Can you work these out from the model? Positions are in its coordinate system, mm. Face numbers are marked on the shaded views. A direction names the side the tool comes from. Give positions to 0.01 mm unless a question says otherwise; leave off trailing zeros. Loops run counter-clockwise (first coordinate to the right, second up) from the corner with the lowest first, then second, coordinate; pieces in that order, holes last. Notation, with made-up numbers: M -17,45.5 L -2,45.5 A18 ccw -2,67.5 Z; hole C 22.25,49 d1. An arc over 180 degrees is marked long. Use CSV: the item, a comma, the result in double quotes.
Autodesk Inventor part; units mm, degrees
ref_plane "Work Plane2" through (3.35, 0, 0) normal (0, 0, -1) x (1, 0, 0)
ref_plane "YZ Plane" through (0, 0, 0) normal (1, 0, 0) x (0, 1, 0)
ref_plane "XZ Plane" through (0, 0, 0) normal (0, 1, 0) x (-1, 0, 0)
sketch "Sketch1" plane through (0, 0, 0) normal (0, 0, 1) x (1, 0, 0)
  line L0 (1.88, 0) -> (8, 0)
  line L1 (8, 0) -> (8, 2)
  line L2 (8, 2) -> (3.6, 2)
  line L3 (3.6, 2) -> (3.1706, 1.7853)
  line L4 (3.1706, 1.7853) -> (2.2, 1.7853)
  line L5 (0, 3.5) -> (0, 2.11)
  line L6 (0, 2.11) -> (1.0316, 1.5957)
  line L7 (1.0316, 1.5957) -> (1.88, 0)
  line L8 (-1.6, 0) -> (9.6, 0)
  line L9 (0, -0.7) -> (0, 4.2)
  line L10 (0, 3.5) -> (0.4853, 3.5)
  line L11 (0.4853, 3.5) -> (2.2, 1.7853)
  line L12 (3.6, 2) -> (1.9853, 2) construction
  dimension "d1" = 4.4
  dimension "d2" = 4
  dimension "d3" = 3.5706
  dimension "d4" = 4.22
  dimension "d5" = 26.5
  dimension "d6" = 62
  dimension "d7" = 1.88
  dimension "d8" = 0.4294
  dimension "d12" = 7
  dimension "d13" = 45
  dimension "d15" = 8
  dimension "d24" = 2.2
revolve "Body" add sketch "Sketch1" angle 360 about axis through (1.88, 0, 0) along (1, 0, 0) contours L7 L6 L5 L10 L11 L4 L3 L2 L1 L0
sketch "Sketch2" plane through (0, 0, 0) normal (-1, 0, 0) x (0, 0, 1)
  line L0 (0, 2.11) -> (0, 0) construction
  line L1 (0, 0) -> (2.11, 0) construction
  arc A0 (0.633, 0) -> (0, 0.633) centre (0, 0) ccw construction
  arc A1 (0.7385, 0) -> (0, 0.7385) centre (0, 0) ccw construction
  arc A2 (2.0511, 0.495) -> (0.495, 2.0511) centre (0, 0) ccw
  line L2 (0, 0) -> (1.492, 1.492) construction
  line L3 (0.495, 2.0511) -> (0.3793, 0.6337)
  line L4 (2.0511, 0.495) -> (0.6337, 0.3793)
  arc A3 (0.495, 2.0511) -> (0, 2.11) centre (0, 0) ccw
  arc A4 (2.11, 0) -> (2.0511, 0.495) centre (0, 0) ccw
  line L5 (0, -4.9) -> (0, 4.9)
  line L6 (-4.9, 0) -> (4.9, 0)
  arc A5 (0.495, -2.0511) -> (2.0511, -0.495) centre (0, 0) ccw
  line L7 (0.495, -2.0511) -> (0.3793, -0.6337)
  line L8 (2.0511, -0.495) -> (0.6337, -0.3793)
  arc A6 (0, -2.11) -> (0.495, -2.0511) centre (0, 0) ccw
  arc A7 (2.0511, -0.495) -> (2.11, 0) centre (0, 0) ccw
  arc A8 (-0.495, 2.0511) -> (-2.0511, 0.495) centre (0, 0) ccw
  line L9 (-0.495, 2.0511) -> (-0.3793, 0.6337)
  line L10 (-2.0511, 0.495) -> (-0.6337, 0.3793)
  arc A9 (0, 2.11) -> (-0.495, 2.0511) centre (0, 0) ccw
  arc A10 (-2.0511, 0.495) -> (-2.11, 0) centre (0, 0) ccw
  arc A11 (-0.495, -2.0511) -> (0, -2.11) centre (0, 0) ccw
  arc A12 (-2.0511, -0.495) -> (-0.495, -2.0511) centre (0, 0) ccw
  arc A13 (-2.11, 0) -> (-2.0511, -0.495) centre (0, 0) ccw
  line L11 (-2.0511, -0.495) -> (-0.6337, -0.3793)
  line L12 (-0.495, -2.0511) -> (-0.3793, -0.6337)
  arc A14 (0.3793, 0.6337) -> (0.6337, 0.3793) centre (0.6145, 0.6145) ccw
  arc A15 (0.6337, -0.3793) -> (0.3793, -0.6337) centre (0.6145, -0.6145) ccw
  arc A16 (-0.6337, 0.3793) -> (-0.3793, 0.6337) centre (-0.6145, 0.6145) ccw
  arc A17 (-0.3793, -0.6337) -> (-0.6337, -0.3793) centre (-0.6145, -0.6145) ccw
  point P0 (1.492, -1.492)
  point P1 (-1.492, 1.492)
  point P2 (-1.492, -1.492)
  dimension "d17" = 1.266
  dimension "d18" = 1.477
  dimension "d19" = 4.22
  dimension "d20" = 45
  dimension "d21" = 0.495
extrude "Slot" add sketch "Sketch2" against normal up to next draft 5 contours L4 A14 L3 A2 | A5 L7 A15 L8 | L9 A16 L10 A8 | A12 L11 A17 L12
fillet "Fillet1" radius 0.198 4 edges at (0, 2.11, 0) (0, 0, -2.11) (0, -2.11, 0) (0, 0, 2.11)
thread "Thread"
chamfer "Chamfer1" distance 0.4294 distance2 0.2147 1 edges at (8, -2, 0) measured on face at (8, -0.499, 0.4421)
ref_plane "Work Plane2" through (3.35, 0, 0) normal (0, 0, -1) x (1, 0, 0)
equation "\"d17\" = 0.3 * SDM"
equation "\"d18\" = 0.35 * SDM"
equation "\"d19\" = SDM"
equation "\"d21\" = 0.5 * SBR"
equation "\"d1\" = GEL"
equation "\"d2\" = GD"
equation "\"d3\" = BDM"
equation "\"d4\" = SDM"
equation "\"d7\" = INTI"
equation "\"d8\" = GAL"
equation "\"d12\" = KOD"
equation "\"d13\" = 0.5 * SEWI"
equation "\"d15\" = NLG"
equation "\"d24\" = KOH"
equation "\"d23\" = 0.2 * SBR"
equation "\"d10\" = GEL"
equation "\"d25\" = -0.5 * SPD + 0.5 * GD"
equation "\"d26\" = 0.5 * GAL"
equation "\"NLG\" = 8"
equation "\"GEL\" = 4.4"
equation "\"GAL\" = 0.61345 * PTC"
equation "\"SPD\" = NND - 1.2269 * PTC"
equation "\"KOD\" = 7"
equation "\"KOH\" = 2.2"
equation "\"SBR\" = 0.99"
equation "\"INTI\" = 1.88"
equation "\"SDM\" = 4.22"
equation "\"GD\" = NND"
equation "\"BDM\" = NND - GAL"
equation "\"SEWI\" = 90deg"
equation "\"d9\" = SDM"
equation "\"GUL\" = 0.61345 * PTC"
equation "\"TOA\" = 30deg"
equation "\"EPV\" = 4.2"
equation "\"THREADDIA\" = 4"
equation "\"RR\" = 0.4"
equation "\"PTC\" = 0.7"
equation "\"NND\" = 4"
equation "\"GD1\" = THREADDIA - 1.2269 * PTC"
properties part number "AS 1427 - M4 x 8" material "Steel, Mild"
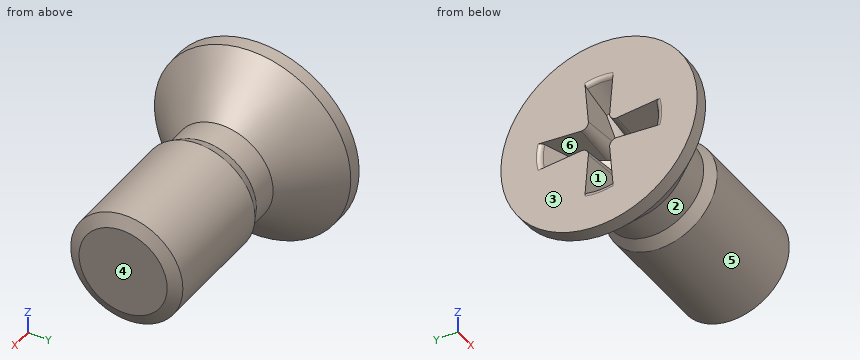
Q1. I want a section at B-B, the plane x = 2.75. Please give me the cut outline in (y, z), then the cut area to 3 significant figures.
Model answer:
outline,"C 0,0 d3.57"
area,"10.0 mm2"
Q2. Please list where these lines run through material, in increasing order: L1, parallel to Y at x = 1.25, z = -0.75; L2, parallel to Z at x = 3.75, y = 0; L3, parallel to Z at x = 0.5, y = 1. Write a range as from..to.
Model answer:
L1,"-2.63..-0.28, 0.28..2.63"
L2,"-2..2"
L3,"-3.34..-0.37, 0.37..3.34"
Q3. If we mould it in two halves opening along Z, with no side actions, what happens to the marked faces 1, 2 and 3? For each: released by +Z, released by -Z, zero draft, split by the parting line, or undercut.
Model answer:
face 1,"undercut"
face 2,"split by the parting line"
face 3,"zero draft"
Q4. I want a section at A-A, the plane x = 5.5. Please give me the cut outline in (y, z), then the cut area to 3 significant figures.
Model answer:
outline,"C 0,0 d4"
area,"12.6 mm2"
Q5. I'm going to push flat-ended pins straight in: P1, Ø1.5, axis at y = 2, z = 0, coming from the +X side; P2, Ø1.5, axis at y = 2, z = -2.5, coming from the +X side; P3, Ø1.5, axis at x = 4.5, z = 1, coming from the +Y side; P4, Ø1.5, axis at x = 2, y = -0.5, coming from the +Z side. Where does each tip first touch, or does it pass through?
Model answer:
P1,"x = 8"
P2,"x = 1.53"
P3,"y = 1.98"
P4,"z = 2.7"
Q6. For the marked faces 4, 5 and 6, which set-ups out of +Z, -Z, +X, -X, +Y, -Y let a thin tool reach every point of the face, with its end or its side?
Model answer:
face 4,"+Z, -Z, +X, +Y, -Y"
face 5,"+X"
face 6,"-X"
